Could you check a few things on this model? Use its own coordinates, in mm. Face numbers are marked on the shaded views. Give positions to 0.01 mm unless a question says otherwise; leave off trailing zeros. Use a Markdown table: item, result. Add a question column.
Item 1: If I drill on L1, parallel to Y at x = 24.75, z = 0; L2, parallel to Y at x = -14.5, z = -4.5; L3, parallel to Z at x = 14, y = 13, over which ranges is the centre line in solid material (lowest first)? Write a range as from..to.
Item 2: If we mould it in two halves opening along Y, with no side actions, what happens to the marked faces 1 and 2? For each: released by +Y, released by -Y, zero draft, split by the parting line, or undercut.
Item 3: I'm going to push flat-ended pins straight in: pin 1 Ø10 at (x, y) = (2.5, 20.5) entering from +Z; pin 2 Ø8 at (x, z) = (-5.5, -7.5) entering from +Y; pin 3 Ø3 at (x, y) = (7.5, -15.5) entering from -Z. Where does each tip first touch, or does it pass through?
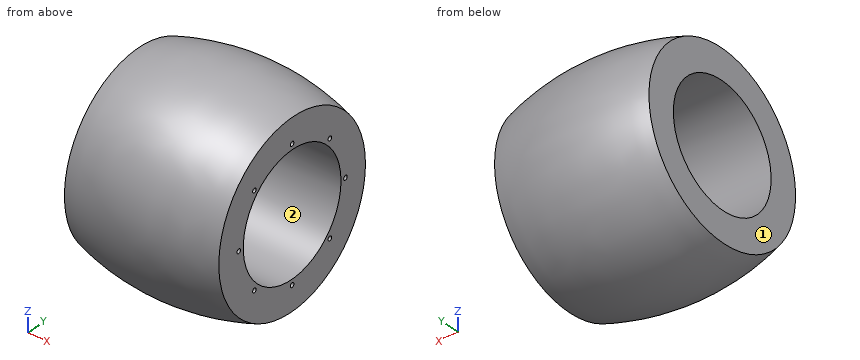
from build123d import *

# Parameters (mm, degrees)
FORMSENKUNG_F_R_M3_SENKSCHRAUBE_MIT_INNE_D           = 1.6
FORMSENKUNG_F_R_M3_SENKSCHRAUBE_MIT_INNE_DEPTH       = 12.5
FORMSENKUNG_F_R_M3_SENKSCHRAUBE_MIT_INNE_CSINK_D     = 3.75
FORMSENKUNG_F_R_M3_SENKSCHRAUBE_MIT_INNE_CSINK_ANGLE = 90
FORMSENKUNG_F_R_M3_SENKSCHRAUBE_MIT_INNE_TIP         = 0.480688495


with BuildPart() as part:
    # Skizze1 → Rotation1 (revolve)
    with BuildSketch(Plane.XY):
        with BuildLine():
            ThreePointArc((26, 29.304134332), (25.393087675, 31.113314086), (23.817912414, 32.190484845))
            ThreePointArc((23.817912414, 32.190484845), (0, 35.5), (-23.817912414, 32.190484845))
            ThreePointArc((-23.817912414, 32.190484845), (-25.393087675, 31.113314086), (-26, 29.304134332))
            Line((-26, 29.304134332), (-26, 22))
            Line((-26, 22), (-28, 22))
            Line((-28, 22), (-28, 33))
            ThreePointArc((-28, 33), (0, 37.5), (28, 33))
            Line((28, 33), (28, 22))
            Line((28, 22), (26, 22))
            Line((26, 22), (26, 29.304134332))
        make_face()
        with BuildLine():
            Line((26, 22), (26, 29.304134332))
            ThreePointArc((26, 29.304134332), (25.393087675, 31.113314086), (23.817912414, 32.190484845))
            ThreePointArc((23.817912414, 32.190484845), (0, 35.5), (-23.817912414, 32.190484845))
            ThreePointArc((-23.817912414, 32.190484845), (-25.393087675, 31.113314086), (-26, 29.304134332))
            Line((-26, 29.304134332), (-26, 22))
            Line((-26, 22), (26, 22))
        make_face()
    revolve(axis=Axis((0, 0, 0), (-1, 0, 0)))

    # Formsenkung f_r M3 Senkschraube mit Inne
    with Locations(Plane(origin=(32.5, -4.747521164, 0), x_dir=(0, 0, 1), z_dir=(1, 0, 0))):
        with Locations((0, -28.747521164), (16.970562748, -21.718083913), (24, -4.747521164), (16.970562748, 12.223041584), (0, 19.252478836), (-16.970562748, 12.223041584), (-24, -4.747521164), (-16.970562748, -21.718083913), (0, -4.747521164)):
            CounterSinkHole(FORMSENKUNG_F_R_M3_SENKSCHRAUBE_MIT_INNE_D / 2, FORMSENKUNG_F_R_M3_SENKSCHRAUBE_MIT_INNE_CSINK_D / 2, depth=FORMSENKUNG_F_R_M3_SENKSCHRAUBE_MIT_INNE_DEPTH, counter_sink_angle=FORMSENKUNG_F_R_M3_SENKSCHRAUBE_MIT_INNE_CSINK_ANGLE)
            with Locations((0, 0, -(FORMSENKUNG_F_R_M3_SENKSCHRAUBE_MIT_INNE_DEPTH + FORMSENKUNG_F_R_M3_SENKSCHRAUBE_MIT_INNE_TIP / 2))):  # 118° drill point
                Cone(0, FORMSENKUNG_F_R_M3_SENKSCHRAUBE_MIT_INNE_D / 2, FORMSENKUNG_F_R_M3_SENKSCHRAUBE_MIT_INNE_TIP, mode=Mode.SUBTRACT)


solid = part.part
Findings below:
| question | item | result |
|---|---|---|
| 1 | L1 | y = -34..-24.8, -23.2..-22, 22..23.2, 24.8..34 |
| 1 | L2 | y = -36.04..-21.53, 21.53..36.04 |
| 1 | L3 | z = -34..-17.75, 17.75..34 |
| 2 | face 1 | zero draft |
| 2 | face 2 | undercut |
| 3 | pin 1 | stops at z = 34.11 |
| 3 | pin 2 | stops at y = 37.22 |
| 3 | pin 3 | stops at z = -34.46 |
